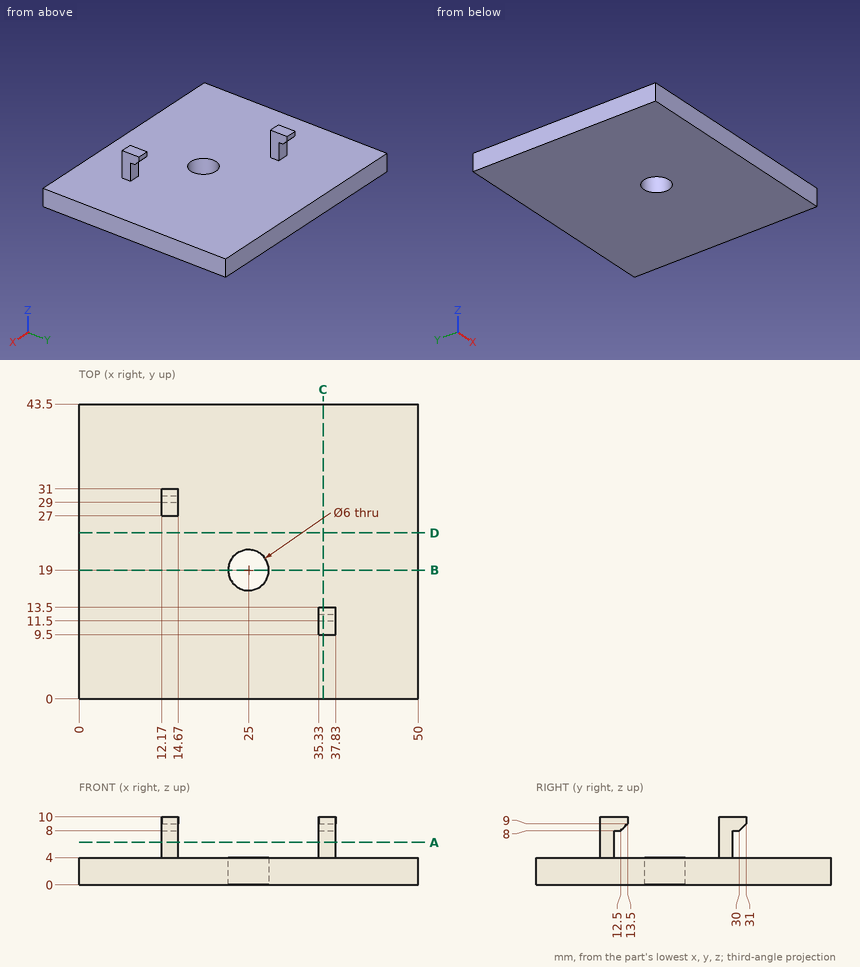
Input: dimensioned drawing with shaded views. Units: mm. Origin: part minimum x, y, z. Coordinates: 2 decimals unless noted, no trailing zeros. Loops run counter-clockwise (first coordinate to the right, second up) from the corner with the lowest first, then second, coordinate; pieces in that order, holes last. Notation, with made-up numbers: M -25,-4 L 34,-4 A23 cw 34,33 Z; hole C 57,4 d9. An arc over 180 degrees is marked long. Use a Markdown table: item, result. Add a question column.
1) Section A-A, the plane z = 6.25. Return the cut outline in (x, y).
2) Section D-D, the plane y = 24.5. Return the cut outline in (x, z).
3) Section B-B, the plane y = 19. Return the cut outline in (x, z), plus the area to 3 significant figures.
4) Line query: L1, parallel to Y at x = 25, z = 1.95; L2, parallel to Z at x = 19, y = 37.5; L3, parallel to X at y = 17, z = 1.5. Output: solid intervals per line, ascending. Write a range as from..to.
5) Section C-C, the plane x = 36. Return the cut outline in (y, z).
6) Pin query (flat end, axial travel): P1, Ø3, axis at y = 28.5, z = 7, coming from the -X side; P2, Ø2, axis at y = 29.5, z = 5.5, coming from the +X side; P3, Ø0.8, axis at x = 14, z = 7.5, coming from the -Y side; P4, Ø1.5, axis at x = 41.5, z = 6, coming from the -Y side. Return the tip coordinate at first contact, or that it passes through.
Answer below:
| question | item | result |
|---|---|---|
| 1 | outline | M 12.17,27 L 14.67,27 L 14.67,29 L 12.17,29 Z; M 35.33,9.5 L 37.83,9.5 L 37.83,11.5 L 35.33,11.5 Z |
| 2 | outline | M 0,0 L 50,0 L 50,4 L 0,4 Z |
| 3 | outline | M 0,0 L 22,0 L 22,4 L 0,4 Z; M 28,0 L 50,0 L 50,4 L 28,4 Z |
| 3 | area | 176 mm2 |
| 4 | L1 | 0..16, 22..43.5 |
| 4 | L2 | 0..4 |
| 4 | L3 | 0..22.76, 27.24..50 |
| 5 | outline | M 0,0 L 43.5,0 L 43.5,4 L 11.5,4 L 11.5,8 L 12.5,8 L 13.5,9 L 13.5,10 L 9.5,10 L 9.5,4 L 0,4 Z |
| 6 | P1 | x = 12.17 |
| 6 | P2 | x = 14.67 |
| 6 | P3 | y = 27 |
| 6 | P4 | through |
